The listing builds one solid part. Answer for the finished solid, in the listing's coordinates (mm). Face numbers are marked on the shaded views. A direction names the side the tool comes from. Round coordinates to 2 decimals unless told otherwise and drop trailing zeros. Loops run counter-clockwise (first coordinate to the right, second up) from the corner with the lowest first, then second, coordinate; pieces in that order, holes last. Notation, with made-up numbers: (23.5, 33.25) -> (53.5, 33.25) arc R16 ccw to (53.5, 56.25) -> close; hole circle Ø8 at (41, 26). An arc over 180 degrees is marked (long way). Write each question's results on one line, items separated by ' | '. Start each with the question number.
(1) For the marked faces 1 and 2, determine the directions among +Z, -Z, +X, -X, +Y, -Y from which every point of the face is accessible in a straight line to the end or side of a thin tool.
(2) A flat-ended cylindrical pin translates along its axis: pin 1 (10 mm diameter, centred on x = 25, z = 11.5, fed in from +Y). Find the tip coordinate at first contact, or state that the pin passes through.
(3) The part is cut by section A-A (z = 14.5). Determine the outline of the cut face in (x, y).
(4) Straight lines are drawn through the part: probe 1 along Y at (x, z) = (25.5, 11.5); probe 2 along X at (y, z) = (6.5, 15.75); probe 3 along X at (y, z) = (0.75, 9.5). For each, find the intervals that lie inside material, in ascending order.
(5) The part is cut by section B-B (x = 33). Determine the outline of the cut face in (y, z).
```python
from build123d import *

# Parameters (mm, degrees)
BOSS_EXTRUDE1_DEPTH = 20.32
FILLET1_R           = 1.27


with BuildPart() as part:
    # Sketch1 → Boss-Extrude1 (new body)
    with BuildSketch(Plane.XY):
        Polygon((0, 0), (0, 10.16), (18.531128405, 10.16), (20.968059336, 7.62), (38.1, 7.62), (38.1, 0), align=None)
    extrude(amount=BOSS_EXTRUDE1_DEPTH)

    # Fillet1
    fillet1_edges = [part.edges().sort_by_distance(p)[0] for p in [
        (29.534029668, 7.62, 20.32),
        (0, 0, 10.16),
        (0, 10.16, 10.16),
        (18.531128405, 10.16, 10.16),
        (20.968059336, 7.62, 10.16),
        (38.1, 7.62, 10.16),
        (38.1, 0, 10.16),
        (19.74959387, 8.89, 20.32),
        (9.265564202, 10.16, 20.32),
        (0, 5.08, 20.32),
        (19.05, 0, 20.32),
        (0, 5.08, 0),
        (9.265564202, 10.16, 0),
        (19.74959387, 8.89, 0),
        (38.1, 3.81, 20.32),
        (29.534029668, 7.62, 0),
        (38.1, 3.81, 0),
        (19.05, 0, 0),
    ]]
    fillet(fillet1_edges, radius=FILLET1_R)


solid = part.part
```
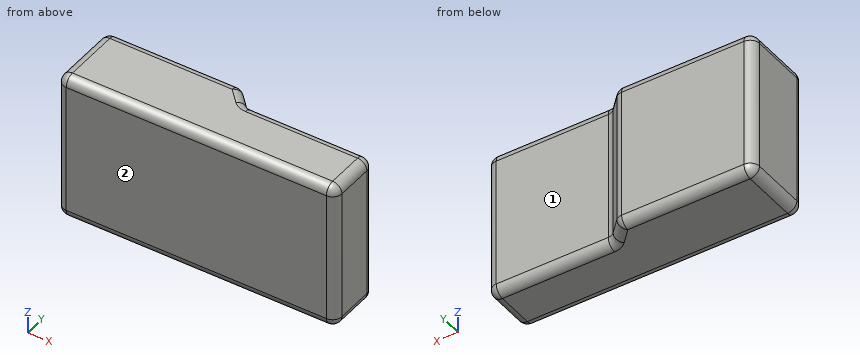
Checked values:
1) face 1: +Z, -Z, +X, +Y | face 2: +Z, -Z, +X, -X, -Y
2) pin 1: stops at y = 8.63
3) outline: (0, 1.27) arc R1.27 ccw to (1.27, 0) -> (36.83, 0) arc R1.27 ccw to (38.1, 1.27) -> (38.1, 6.35) arc R1.27 ccw to (36.83, 7.62) -> (21.51, 7.62) arc R1.27 cw to (20.59, 8.01) -> (18.91, 9.77) arc R1.27 ccw to (17.99, 10.16) -> (1.27, 10.16) arc R1.27 ccw to (0, 8.89) -> close
4) probe 1: y = 0 to 7.62 | probe 2: x = 0 to 38.09 | probe 3: x = 0.11 to 37.99
5) outline: (0, 1.27) arc R1.27 ccw to (1.27, 0) -> (6.35, 0) arc R1.27 ccw to (7.62, 1.27) -> (7.62, 19.05) arc R1.27 ccw to (6.35, 20.32) -> (1.27, 20.32) arc R1.27 ccw to (0, 19.05) -> close
